from build123d import *

# Parameters (mm, degrees)
SKETCH2_R          = 1.5
CUT_EXTRUDE1_DEPTH = 8


with BuildPart() as part:
    # Sketch1 → Revolve1 (revolve)
    with BuildSketch(Plane.XY):
        with BuildLine():
            Line((0, 0), (-3.25, 0))
            Line((-3.25, 0), (-3.25, 1))
            Line((-3.25, 1), (-1.658312395, 1))
            Line((-1.658312395, 1), (-1.658312395, 2))
            ThreePointArc((-1.658312395, 2), (-3, 4.5), (-1.658312395, 7))
            Line((-1.658312395, 7), (0, 7))
            Line((0, 7), (0, 0))
        make_face()
    revolve(axis=Axis((0, 0, 0), (0, 1, 0)))

    # Sketch2 → Cut-Extrude1 (cut, through all)
    with BuildSketch(Plane(origin=(0, 7, 0), x_dir=(1, 0, 0), z_dir=(0, 1, 0))):
        Circle(SKETCH2_R)
    extrude(amount=-CUT_EXTRUDE1_DEPTH, mode=Mode.SUBTRACT)


solid = part.part
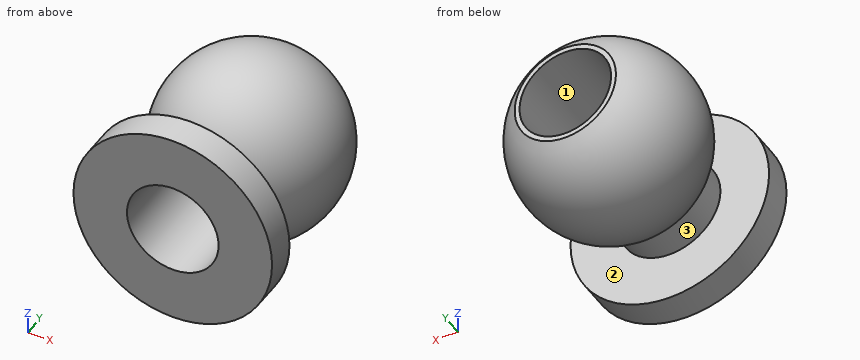
Design review of the part built by this model. Coordinates are the model's own, in mm. Face numbers are marked on the shaded views. Give positions to 0.01 mm unless a question says otherwise; leave off trailing zeros. Loops run counter-clockwise (first coordinate to the right, second up) from the corner with the lowest first, then second, coordinate; pieces in that order, holes last. Notation, with made-up numbers: M 10,52.5 L 18,52.5 A29 ccw 18,78.5 Z; hole C 43.5,-39.75 d11. An arc over 180 degrees is marked long. One line per question, with ' | ' between items. Start each with the question number.
1. To check wall thickness, follow L1, parallel to Y at x = 2.5, z = -1.25; L2, parallel to Y at x = -2, z = -0.75; L3, parallel to Z at x = 0, y = 4.25. State the ranges of each line that lie inside material, in increasing order.
2. Add section B-B (z = 0.75). Write out the cut boundary in (x, y).
3. Insertion check: P1, Ø1.8, axis at x = 0, z = 0, coming from the +Y side (3 decimals); P2, Ø1, axis at x = -1, y = 4.5, coming from the +Z side; P3, Ø3, axis at y = 1.5, z = -2, coming from the -X side; P4, Ø1, axis at y = 3.5, z = -1.5, coming from the +X side. Each pin has a flat end and moves straight along its axis. Give the tip position at first contact, or say it passes through.
4. Add section D-D (z = 2.5). Write out the cut boundary in (x, y), plus the area to 3 significant figures.
5. Add section C-C (y = 6.75). Write out the cut boundary in (x, z), plus the area to 3 significant figures.
6. The part is to be moulded in two halves that separate along X. For the marked faces 1, 2 and 3, say which applies: released by +X, released by -X, zero draft, split by the parting line, or undercut.
7. Add section A-A (x = 0). Write out the cut boundary in (y, z).
Worked out:
1) L1: y = 0 to 1, 3.41 to 5.59 | L2: y = 0 to 1, 2.39 to 6.61 | L3: z = -2.99 to -1.5, 1.5 to 2.99
2) outline: M -3.16,0 L -1.3,0 L -1.3,7 L -1.48,7 A2.9 ccw -1.48,2 L -1.48,1 L -3.16,1 Z; M 1.3,0 L 3.16,0 L 3.16,1 L 1.48,1 L 1.48,2 A2.9 ccw 1.48,7 L 1.3,7 Z
3) P1: passes through | P2: stops at z = 2.96 | P3: stops at x = -3.2 | P4: stops at x = 2.7
4) outline: M -2.08,0 L 2.08,0 L 2.08,1 L -2.08,1 Z; C 0,4.5 d3.32 | area: 12.8 mm²
5) outline: C 0,0 d3.97; hole C 0,0 d3 | area: 5.30 mm²
6) face 1: undercut | face 2: zero draft | face 3: split by the parting line
7) outline: M 0,-3.25 L 1,-3.25 L 1,-1.66 L 2,-1.66 A3 ccw 7,-1.66 L 7,-1.5 L 0,-1.5 Z; M 0,1.5 L 7,1.5 L 7,1.66 A3 ccw 2,1.66 L 1,1.66 L 1,3.25 L 0,3.25 Z
